CAD build for the part. Positions are in the model's coordinates, mm. A direction names the side the tool comes from. Coordinates: 2 decimals unless noted, no trailing zeros. Order: outer loops, then holes, each group sorted by start corner. A loop starts at its lowest first (then second) coordinate and runs counter-clockwise, first axis right, second up. Notation, with made-up numbers: (40.5, 31.5) - (84.5, 31.5) arc R12 cw to (84.5, 44.5) - close; hole circle Ø5 at (22.5, 16.25). An arc over 180 degrees is marked (long way). Return JSON: item names as keys, results as strings.
from build123d import *

# Parameters (mm, degrees)
F1_DEPTH = 25
F2_DEPTH = 37.6
F3_DEPTH = 25
F4_DEPTH = 25
F5_DEPTH = 25


with BuildPart() as f1:
    # F0 (on Front) → F1 (new body)
    with BuildSketch(Plane.XZ):
        Polygon((60, -27.5), (60, 27.5), (-60, 27.5), (-60, 14.1944857314), (-90.527780354, 14.1944857314), (-90, -27.5), (-60, -27.5), (35, -27.5), align=None)
        with BuildLine():
            ThreePointArc((-58.75, -19.5), (-59.1161165235, -20.3838834765), (-60, -20.75))
            ThreePointArc((-60, -20.75), (-60.8838834765, -18.6161165235), (-58.75, -19.5))
        make_face(mode=Mode.SUBTRACT)
        with BuildLine():
            ThreePointArc((36.25, -19.5), (35.8838834765, -20.3838834765), (35, -20.75))
            ThreePointArc((35, -20.75), (34.1161165235, -18.6161165235), (36.25, -19.5))
        make_face(mode=Mode.SUBTRACT)
    extrude(amount=F1_DEPTH)

    # F0 (on Front) → F2 (join)
    with BuildSketch(Plane.XZ):
        Polygon((60, -27.5), (60, 27.5), (-60, 27.5), (-60, 14.1944857314), (-90.527780354, 14.1944857314), (-90, -27.5), (-60, -27.5), (35, -27.5), align=None)
        with BuildLine():
            ThreePointArc((-58.75, -19.5), (-59.1161165235, -20.3838834765), (-60, -20.75))
            ThreePointArc((-60, -20.75), (-60.8838834765, -18.6161165235), (-58.75, -19.5))
        make_face(mode=Mode.SUBTRACT)
        with BuildLine():
            ThreePointArc((36.25, -19.5), (35.8838834765, -20.3838834765), (35, -20.75))
            ThreePointArc((35, -20.75), (34.1161165235, -18.6161165235), (36.25, -19.5))
        make_face(mode=Mode.SUBTRACT)
    extrude(amount=F2_DEPTH)

    # F0 (on Front) → F3 (join)
    with BuildSketch(Plane.XZ):
        Polygon((60, -27.5), (60, 27.5), (-60, 27.5), (-60, 14.1944857314), (-90.527780354, 14.1944857314), (-90, -27.5), (-60, -27.5), (35, -27.5), align=None)
        with BuildLine():
            ThreePointArc((-58.75, -19.5), (-59.1161165235, -20.3838834765), (-60, -20.75))
            ThreePointArc((-60, -20.75), (-60.8838834765, -18.6161165235), (-58.75, -19.5))
        make_face(mode=Mode.SUBTRACT)
        with BuildLine():
            ThreePointArc((36.25, -19.5), (35.8838834765, -20.3838834765), (35, -20.75))
            ThreePointArc((35, -20.75), (34.1161165235, -18.6161165235), (36.25, -19.5))
        make_face(mode=Mode.SUBTRACT)
    extrude(amount=F3_DEPTH)

    # F4 (add): a face of the model
    f4_faces = [f1.faces().sort_by_distance(p)[0] for p in [
        (-12.0583061009, -37.6, -1.0349945088),
    ]]
    extrude(f4_faces, amount=F4_DEPTH)

    # F0 (on Front) → F5 (join)
    with BuildSketch(Plane.XZ):
        Polygon((60, -27.5), (60, 27.5), (-60, 27.5), (-60, 14.1944857314), (-90.527780354, 14.1944857314), (-90, -27.5), (-60, -27.5), (35, -27.5), align=None)
        with BuildLine():
            ThreePointArc((-58.75, -19.5), (-59.1161165235, -20.3838834765), (-60, -20.75))
            ThreePointArc((-60, -20.75), (-60.8838834765, -18.6161165235), (-58.75, -19.5))
        make_face(mode=Mode.SUBTRACT)
        with BuildLine():
            ThreePointArc((36.25, -19.5), (35.8838834765, -20.3838834765), (35, -20.75))
            ThreePointArc((35, -20.75), (34.1161165235, -18.6161165235), (36.25, -19.5))
        make_face(mode=Mode.SUBTRACT)
    extrude(amount=F5_DEPTH)


solid = f1.part
Item 1: Wall check: L1, parallel to X at y = -19, z = -19.5; L2, parallel to X at y = -30, z = -19; L3, parallel to Z at x = 35, y = -41.5. Give the ranges that are in metal, low to high. Write a range as [from, to].
Findings below:
{"L1": "x = [-90.1, -61.25], [-58.75, 33.75], [36.25, 60]", "L2": "x = [-90.11, -61.15], [-58.85, 33.85], [36.15, 60]", "L3": "z = [-27.5, -20.75], [-18.25, 27.5]"}
Item 2: Band-saw the part on C-C, the plane z = 23. List the corners of the cut face in (x, y).
Findings below:
{"outline": "(-60, -62.6) - (60, -62.6) - (60, 0) - (-60, 0) - close"}
Item 3: Band-saw the part on B-B, the plane x = -68. List the corners of the cut face in (y, z), then the cut area to 3 significant figures.
Findings below:
{"outline": "(-62.6, -27.5) - (0, -27.5) - (0, 14.19) - (-62.6, 14.19) - close", "area": "2,610 mm²"}
Item 4: Band-saw the part on A-A, the plane y = -45.5. List the corners of the cut face in (x, z).
Findings below:
{"outline": "(-90.53, 14.19) - (-90, -27.5) - (60, -27.5) - (60, 27.5) - (-60, 27.5) - (-60, 14.19) - close; hole circle Ø2.5 at (-60, -19.5); hole circle Ø2.5 at (35, -19.5)"}
Item 5: Which spindle directions (+Z, -Z, +X, -X, +Y, -Y) get a long thin tool onto all of the face, cutting with end or side? Do faces 1 (the flat face through (-60, -31, 21)), 2 (the flat face through (-16, -31, -27.5)). Say none if no direction does.
Findings below:
{"face 1": "+Z, -X, +Y, -Y", "face 2": "-Z, +X, -X, +Y, -Y"}
Item 6: Drop flat-ended pins along their axis: P1, Ø15.5, axis at x = -68, y = -36, coming from the +Z side; P2, Ø1.5, axis at y = -47, z = -16.5, coming from the -X side. Give the stop position or say it passes through.
Findings below:
{"P1": "stops at z = 14.19", "P2": "stops at x = -90.15"}
